Build history of the part. All positions in model axes, mm. A direction names the side the tool comes from. Give positions to 0.01 mm unless a question says otherwise; leave off trailing zeros. Write each loop counter-clockwise with the first axis right and the second up, starting at its lowest first coordinate (ties: lowest second). Pieces come first, ordered by that corner, then holes. Notation, with made-up numbers: (1.25, -12) -> (8.25, -12) arc R24 cw to (8.25, -1) -> close; hole circle Ø1 at (-13, -9). An arc over 180 degrees is marked (long way). One line per question, with ' | ' between items. Start each with the question number.
(1) Band-saw the part on A-A, the plane y = 31. Give the cut face in (x, z) (3 decimals).
(2) Pin check, flat tips, straight feed: P1, Ø1, axis at y = 59, z = -16, coming from the +X side; P2, Ø2, axis at y = 27.5, z = -9.5, coming from the +X side; P3, Ø0.5, axis at x = 19, z = -18, coming from the +Y side. Stop position of each tip, or through.
(3) Pull direction Y, two halves, no side cores. Call faces 3 (the cylindrical face through (-4.6, 9.7, -8.6)), 4 (the cylindrical face through (9.12, 30.934, -21.274)), 5 (the flat face through (9, 31, -22)): released by +Y, released by -Y, zero draft, split by the parting line, or undercut.
(4) Band-saw the part on D-D, the plane z = -11. Give the cut face in (x, y), and give its area (3 significant figures).
(5) Band-saw the part on B-B, the plane z = -1.75. Give the cut face in (x, y).
(6) Tool access for faces 1 (the flat face through (9, 63, -11)), 2 (the cylindrical face through (22.9, 9.7, -8.6)): list every direction of +Z, -Z, +X, -X, +Y, -Y with a clear straight run to the whole face (end or side of a thin tool).
(7) Band-saw the part on C-C, the plane y = 11.5. Give the cut face in (x, z).
(8) Drill centre lines: probe 1 along X at (y, z) = (36, -14); probe 2 along Z at (x, y) = (9.5, 32); probe 3 along Y at (x, z) = (13.5, -1.5). Where is each one in solid material? Low to high. Write a range as from..to.
from build123d import *

# Parameters (mm, degrees)
ESQUISSE1_W             = 22
ESQUISSE1_H             = 63
ESQUISSE1_R             = 1.5
BOSS_EXTRU_1_DEPTH      = 18.5
BOSS_EXTRU_2_DEPTH      = 9
BOSS_EXTRU_2_DEPTH_BACK = 27.5
ESQUISSE2_R             = 3
ESQUISSE3_W             = 4
ESQUISSE3_H             = 2
BOSS_EXTRU_3_DEPTH      = 1


with BuildPart() as part:
    # Esquisse1 → Boss.-Extru.1 (new body)
    with BuildSketch(Plane(origin=(0, 0, 0), x_dir=(0, 0, -1), z_dir=(1, 0, 0))):
        with Locations((11, 31.5)):
            Rectangle(ESQUISSE1_W, ESQUISSE1_H)
        with Locations((2.225, 31)):
            Circle(ESQUISSE1_R, mode=Mode.SUBTRACT)
        with Locations(Location((19.775, 31, 0), (0, 0, 180))):
            Circle(ESQUISSE1_R, mode=Mode.SUBTRACT)
    extrude(amount=BOSS_EXTRU_1_DEPTH)

    # Esquisse2 → Boss.-Extru.2 (add, two sides: drawn at the far end of the back side and taken through both)
    with BuildSketch(Plane(origin=(18.5, 0, 0), x_dir=(0, 0, -1), z_dir=(1, 0, 0)).offset(-BOSS_EXTRU_2_DEPTH_BACK)):
        with Locations((11, 11.5)):
            Circle(ESQUISSE2_R)
    extrude(amount=BOSS_EXTRU_2_DEPTH + BOSS_EXTRU_2_DEPTH_BACK)

    # Esquisse3 → Boss.-Extru.3 (add)
    with BuildSketch(Plane(origin=(18.5, 0, 0), x_dir=(0, 0, -1), z_dir=(1, 0, 0))):
        with Locations((5, 59)):
            Rectangle(ESQUISSE3_W, ESQUISSE3_H)
        with Locations((17, 59)):
            Rectangle(ESQUISSE3_W, ESQUISSE3_H)
    extrude(amount=BOSS_EXTRU_3_DEPTH)


solid = part.part
Results:
1) outline: (0, -22) -> (18.5, -22) -> (18.5, -21.275) -> (0, -21.275) -> close; (0, -18.275) -> (18.5, -18.275) -> (18.5, -3.725) -> (0, -3.725) -> close; (0, -0.725) -> (18.5, -0.725) -> (18.5, 0) -> (0, 0) -> close
2) P1: stops at x = 19.5 | P2: stops at x = 18.5 | P3: stops at y = 60
3) face 3: split by the parting line | face 4: undercut | face 5: zero draft
4) outline: (-9, 8.5) -> (0, 8.5) -> (0, 0) -> (18.5, 0) -> (18.5, 8.5) -> (27.5, 8.5) -> (27.5, 14.5) -> (18.5, 14.5) -> (18.5, 63) -> (0, 63) -> (0, 14.5) -> (-9, 14.5) -> close | area: 1,270 mm²
5) outline: (0, 0) -> (18.5, 0) -> (18.5, 29.58) -> (0, 29.58) -> close; (0, 32.42) -> (18.5, 32.42) -> (18.5, 63) -> (0, 63) -> close
6) face 1: +Z, -Z, +X, -X, +Y | face 2: +X
7) outline: (-9, -14) -> (0, -14) -> (0, -22) -> (18.5, -22) -> (18.5, -14) -> (27.5, -14) -> (27.5, -8) -> (18.5, -8) -> (18.5, 0) -> (0, 0) -> (0, -8) -> (-9, -8) -> close
8) probe 1: x = 0..18.5 | probe 2: z = -22..-20.89, -18.66..-3.34, -1.11..0 | probe 3: y = 0..29.69, 32.31..63
